Geometry check sheet. Reference: the model listing, model coordinates, mm. Face numbers are marked on the shaded views. Give positions to 0.01 mm unless a question says otherwise; leave off trailing zeros. Loops run counter-clockwise (first coordinate to the right, second up) from the corner with the lowest first, then second, coordinate; pieces in that order, holes last. Notation, with made-up numbers: (-18, -15.75) -> (39, -15.75) arc R11 ccw to (39, -1.75) -> close; hole circle Ø4 at (40, 68.25). An arc over 180 degrees is marked (long way). Write item = value, one per line.
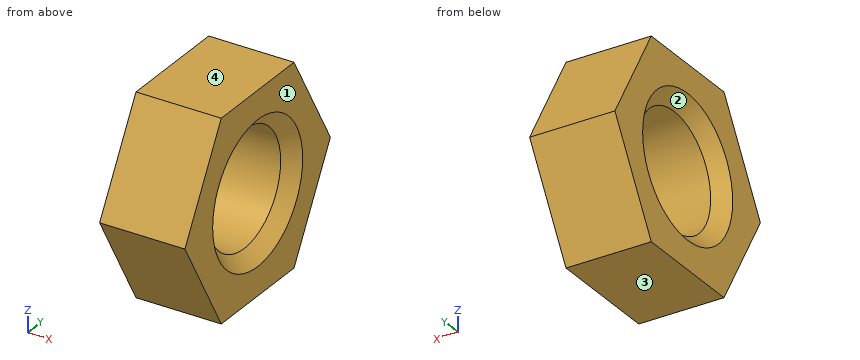
Autodesk Inventor part; units mm, degrees
ref_plane "cp_XY" through (0, 0, 0) normal (1, 0, 0) x (0, 0, -1)
ref_plane "cp_YZ" through (0, 0, 0) normal (0, 0, -1) x (0, 1, 0)
ref_plane "cp_ZX" through (0, 0, 0) normal (0, 1, 0) x (1, 0, 0)
sketch "Sketch_5" plane through (0, 0, 0) normal (0, 0, 1) x (1, 0, 0)
  line L0 (1.5, 0) -> (-1.5, 0)
  line L1 (-1.5, 0) -> (-1.5, 4.375)
  line L2 (-1.5, 4.375) -> (-1.1031, 5.0625)
  line L3 (-1.1031, 5.0625) -> (1.1031, 5.0625)
  line L4 (1.1031, 5.0625) -> (1.5, 4.375)
  line L5 (1.5, 4.375) -> (1.5, 0)
  line L6 (1.5, 0) -> (-1.5, 0)
  dimension "d8" = 3
revolve "Revolution1" add sketch "Sketch_5" angle 360 about axis through (1.5, 0, 0) along (1, 0, 0)
sketch "Sketch_6" plane through (0, 0, 0) normal (0, 0, 1) x (1, 0, 0)
  line L0 (1.5, 0) -> (-1.5, 0)
  line L1 (-1.5, 0) -> (-1.5, 2.5)
  line L2 (-1.5, 2.5) -> (-1.0262, 2.0262)
  line L3 (-1.0262, 2.0262) -> (1.0263, 2.0262)
  line L4 (1.0263, 2.0262) -> (1.5, 2.5)
  line L5 (1.5, 2.5) -> (1.5, 0)
  line L6 (1.5, 0) -> (-1.5, 0)
  line L7 (0, 2.0262) -> (0, 0)
  line L8 (0, 0) -> (0, 9.277)
  dimension "d10" = 3
revolve "Revolution2" cut sketch "Sketch_6" angle 360 about axis through (1.5, 0, 0) along (1, 0, 0)
thread "Thread1"
sketch "Sketch_7" plane through (0, 0, 0) normal (1, 0, 0) x (0, 1, 0)
  line L0 (-7, 7) -> (-7, -7)
  line L1 (-7, -7) -> (7, -7)
  line L2 (7, -7) -> (7, 7)
  line L3 (7, 7) -> (-7, 7)
  line L4 (-2.0207, 3.5) -> (-4.0415, 0)
  line L5 (-4.0415, 0) -> (-2.0207, -3.5)
  line L6 (-2.0207, -3.5) -> (2.0207, -3.5)
  line L7 (2.0207, -3.5) -> (4.0415, 0)
  line L8 (4.0415, 0) -> (2.0207, 3.5)
  line L9 (2.0207, 3.5) -> (-2.0207, 3.5)
extrude "Extrusion1" cut sketch "Sketch_7" along normal mid plane 3
ref_plane "cp_XY" through (0, 0, 0) normal (1, 0, 0) x (0, 0, -1)
ref_plane "cp_YZ" through (0, 0, 0) normal (0, 0, -1) x (0, 1, 0)
ref_plane "cp_ZX" through (0, 0, 0) normal (0, 1, 0) x (1, 0, 0)
ref_plane "nut_to_screw_XY" through (1.2, 0, 0) normal (1, 0, 0) x (0, 0, -1)
ref_plane "nut_to_screw_YZ" through (1.2, 0, 0) normal (0, 0, -1) x (0, 1, 0)
ref_plane "nut_to_screw_ZX" through (1.2, 0, 0) normal (0, 1, 0) x (1, 0, 0)
properties part number "SKNTR4"
Item 1: Section check B-B, the plane x = -0.85. Record the cut outline in (y, z).
Answer:
outline = (-4.04, 0) -> (-2.02, -3.5) -> (2.02, -3.5) -> (4.04, 0) -> (2.02, 3.5) -> (-2.02, 3.5) -> close; hole circle Ø4.05 at (0, 0)
Item 2: Draft check along Z on the marked faces 1, 2, 3 and 4. Enter one of: +Z half, -Z half, draft (parallel to the pull), parting line (faces both ways), or undercut.
Answer:
face_1 = draft
face_2 = undercut
face_3 = -Z half
face_4 = +Z half
Item 3: Section check C-C, the plane y = -2.75. Record the cut outline in (x, z), plus the area to 3 significant figures.
Answer:
outline = (-1.5, -2.24) -> (1.5, -2.24) -> (1.5, 2.24) -> (-1.5, 2.24) -> close
area = 13.4 mm^2
Item 4: Section check A-A, the plane y = 0. Record the cut outline in (x, z).
Answer:
outline = (-1.5, -3.5) -> (1.5, -3.5) -> (1.5, -2.5) -> (1.03, -2.03) -> (-1.03, -2.03) -> (-1.5, -2.5) -> close; (-1.5, 2.5) -> (-1.03, 2.03) -> (1.03, 2.03) -> (1.5, 2.5) -> (1.5, 3.5) -> (-1.5, 3.5) -> close
Item 5: Thickness scan on L1, parallel to Z at x = 0.55, y = 0; L2, parallel to Y at x = -0.2, z = -1.5; L3, parallel to Z at x = -0.3, y = 1. Record the ranges inside material, lowest first. Write a range as [from, to].
Answer:
L1 = [-3.5, -2.03], [2.03, 3.5]
L2 = [-3.18, -1.36], [1.36, 3.18]
L3 = [-3.5, -1.76], [1.76, 3.5]
Item 6: Section check D-D, the plane z = -3. Record the cut outline in (x, y), plus the area to 3 significant figures.
Answer:
outline = (-1.5, -2.31) -> (1.5, -2.31) -> (1.5, 2.31) -> (-1.5, 2.31) -> close
area = 13.9 mm^2
